Build history of the part. All positions in model axes, mm. A direction names the side the tool comes from. Give positions to 0.01 mm unless a question says otherwise; leave off trailing zeros. Loops run counter-clockwise (first coordinate to the right, second up) from the corner with the lowest first, then second, coordinate; pieces in that order, holes last. Notation, with made-up numbers: (81.25, 14) -> (123.25, 14) arc R22 ccw to (123.25, 34) -> close; hole circle Ø10 at (-36, -26). An arc over 180 degrees is marked (long way). Answer as a JSON object with one key per item and string values. Group by question number.
Q1. Two-plate mould, pull along Y, no slides. Class faces 3 (the cylindrical face through (0, 38, -1)), 4 (the cylindrical face through (-1.34, -34.11, -14.7)), 5 (the cylindrical face through (0, -39, -2)), 6 (the cylindrical face through (0.33, 29.52, -14.7)): pulls with the +Y half, pulls with the -Y half, needs draft (parallel to the pull), parting line crosses it, or undercut.
Q2. Band-saw the part on B-B, the plane z = -11.5. Write the cut outline in (x, y).
Q3. Band-saw the part on D-D, the plane y = 32. Write the cut outline in (x, z), plus the area to 3 significant figures.
Q4. Tool access for faces 1 (the flat face through (0, 40, -17)), 2 (the flat face through (-12.5, 0, -10)): list every direction of +Z, -Z, +X, -X, +Y, -Y with a clear straight run to the whole face (end or side of a thin tool).
Q5. Drop flat-ended pins along their axis: pin 1 (6.5 mm diameter, centred on x = 0, y = -32, fed in from +Z); pin 2 (10.5 mm diameter, centred on x = 3.5, y = -14, fed in from +Z). Give the stop position or say it passes through.
Q6. Wall check: probe 1 along Y at (x, z) = (0, -7.75); probe 2 along X at (y, z) = (-19, -12.25); probe 3 along Z at (x, y) = (15.5, 0). Give the ranges that are in metal, low to high. Write a range as from..to.
Q7. Band-saw the part on A-A, the plane y = 0. Write the cut outline in (x, z), plus the area to 3 significant figures.
Q8. Band-saw the part on C-C, the plane x = -11. Write the cut outline in (y, z), plus the area to 3 significant figures.
from build123d import *

# Parameters (mm, degrees)
SKETCH1_W               = 60
SKETCH1_H               = 80
BOSS_EXTRUDE1_DEPTH     = 30
SKETCH2_W               = 25
SKETCH2_H               = 50
CUT_EXTRUDE1_DEPTH      = 20
CUT_EXTRUDE3_DEPTH      = 59.309518948
CUT_EXTRUDE3_DEPTH_BACK = 59.309518948
SKETCH4_R               = 4
CUT_EXTRUDE4_DEPTH      = 59.309518948
CUT_EXTRUDE4_DEPTH_BACK = 29
SKETCH5_R               = 2.5
FILLET1_R               = 5


with BuildPart() as part:
    # Sketch1 → Boss-Extrude1 (new body)
    with BuildSketch(Plane.XY):
        Rectangle(SKETCH1_W, SKETCH1_H)
    extrude(amount=-BOSS_EXTRUDE1_DEPTH)

    # Sketch2 → Cut-Extrude1 (cut)
    with BuildSketch(Plane.XY):
        Rectangle(SKETCH2_W, SKETCH2_H)
    extrude(amount=-CUT_EXTRUDE1_DEPTH, mode=Mode.SUBTRACT)

    # Sketch4 → Cut-Extrude3 (cut, two sides: drawn at the far end of the back side and taken through both)
    with BuildSketch(Plane(origin=(0, 0, 0), x_dir=(0, 0, -1), z_dir=(1, 0, 0)).offset(-CUT_EXTRUDE3_DEPTH_BACK)):
        with Locations((20, 0)):
            Circle(SKETCH4_R)
    extrude(amount=CUT_EXTRUDE3_DEPTH + CUT_EXTRUDE3_DEPTH_BACK, mode=Mode.SUBTRACT)

    # Sketch5 → Cut-Extrude4 (cut, two sides: drawn at the far end of the back side and taken through both)
    with BuildSketch(Plane.XY.offset(-CUT_EXTRUDE4_DEPTH_BACK)):
        with Locations(Location((0, 32, 0), (0, 0, 180))):
            Circle(SKETCH5_R)
        with Locations(Location((0, -32, 0), (0, 0, 180))):
            Circle(SKETCH5_R)
    extrude(amount=CUT_EXTRUDE4_DEPTH + CUT_EXTRUDE4_DEPTH_BACK, mode=Mode.SUBTRACT)

    # Fillet1
    fillet1_edges = [part.edges().sort_by_distance(p)[0] for p in [
        (0, -40, 0),
        (-30, 0, 0),
        (0, 40, 0),
        (30, 0, 0),
        (30, -40, -15),
        (-30, -40, -15),
        (-30, 40, -15),
        (30, 40, -15),
    ]]
    fillet(fillet1_edges, radius=FILLET1_R)


solid = part.part
Worked answers:
{
 "1": {"face 3": "pulls with the +Y half", "face 4": "undercut", "face 5": "pulls with the -Y half", "face 6": "undercut"},
 "2": {"outline": "(-30, -35) arc R5 ccw to (-25, -40) -> (25, -40) arc R5 ccw to (30, -35) -> (30, 35) arc R5 ccw to (25, 40) -> (-25, 40) arc R5 ccw to (-30, 35) -> close; hole (-12.5, -25) -> (12.5, -25) -> (12.5, 25) -> (-12.5, 25) -> close; hole circle Ø5 at (0, -32); hole circle Ø5 at (0, 32)"},
 "3": {"outline": "(-30, -30) -> (30, -30) -> (30, -5) arc R5 ccw to (25, 0) -> (2.5, 0) -> (2.5, -29) -> (-2.5, -29) -> (-2.5, 0) -> (-25, 0) arc R5 ccw to (-30, -5) -> close", "area": "1,640 mm2"},
 "4": {"face 1": "+Z, -Z, +X, -X, +Y", "face 2": "+Z"},
 "5": {"pin 1": "z = 0", "pin 2": "z = -20"},
 "6": {"probe 1": "-40..-34.5, -29.5..-25, 25..29.5, 34.5..40", "probe 2": "-30..-12.5, 12.5..30", "probe 3": "-30..-24, -16..0"},
 "7": {"outline": "(-30, -30) -> (30, -30) -> (30, -24) -> (-30, -24) -> close; (-30, -16) -> (-12.5, -16) -> (-12.5, 0) -> (-25, 0) arc R5 ccw to (-30, -5) -> close; (12.5, -16) -> (30, -16) -> (30, -5) arc R5 ccw to (25, 0) -> (12.5, 0) -> close", "area": "909 mm2"},
 "8": {"outline": "(-40, -30) -> (40, -30) -> (40, -5) arc R5 ccw to (35, 0) -> (25, 0) -> (25, -20) -> (4, -20) arc R4 cw to (-4, -20) -> (-25, -20) -> (-25, 0) -> (-35, 0) arc R5 ccw to (-40, -5) -> close", "area": "1,360 mm2"}
}
